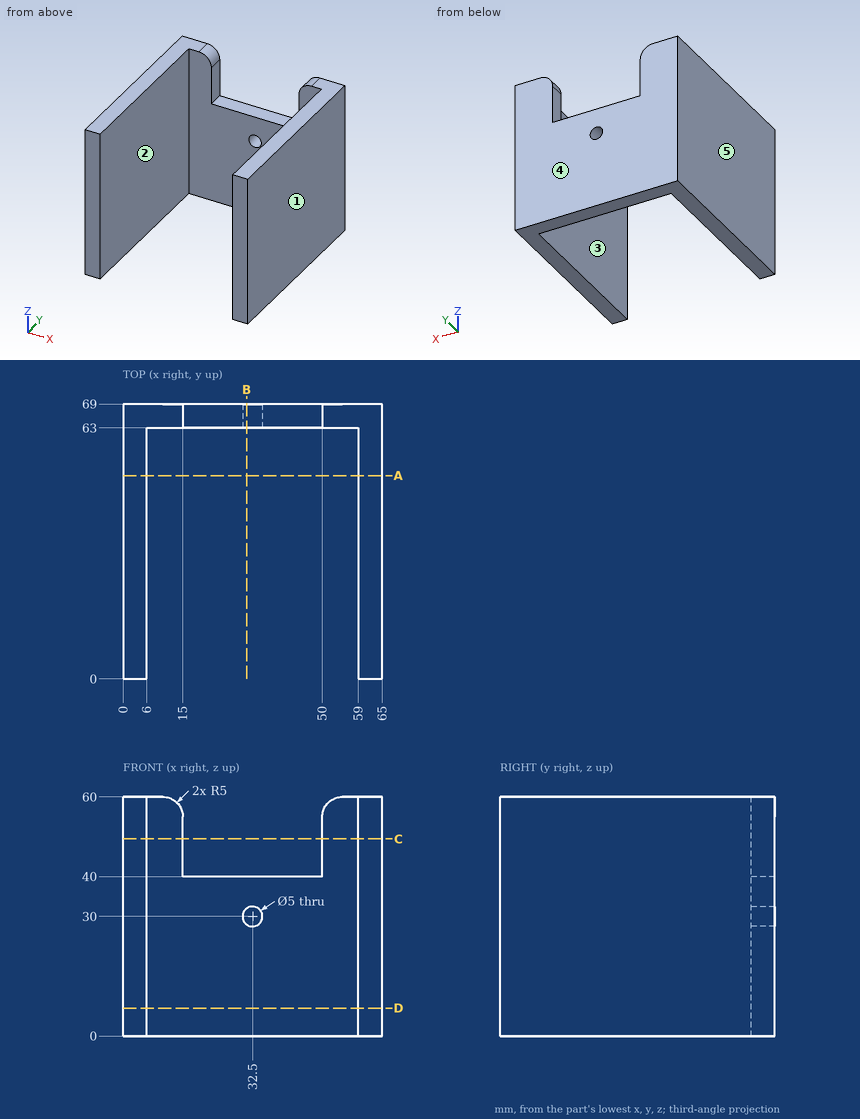
Here's the drawing with two shaded views (mm, measured from the low corner). I have some questions. A direction names the side the tool comes from. Round coordinates to 2 decimals unless told otherwise and drop trailing zeros. Loops run counter-clockwise (first coordinate to the right, second up) from the corner with the lowest first, then second, coordinate; pieces in that order, holes last.
Item 1: Suppose I cut it at C-C, the plane z = 49.5. Write out the boundary of the cut face in (x, y), then the cut area to 3 significant figures.
Item 2: Suppose I cut it at D-D, the plane z = 7. Write out the boundary of the cut face in (x, y).
Item 3: If we mould it in two halves opening along X, with no side actions, what happens to the marked faces 3, 4 and 5? For each: +X half, -X half, draft (parallel to the pull), parting line (faces both ways), or undercut.
Item 4: Which directions (+Z, -Z, +X, -X, +Y, -Y) give clear straight access to the entire face, cutting with the end or side of a thin tool? Please do the marked faces 1 and 2.
Item 5: Please list where these lines run through material, in increasing order: L1, parallel to X at y = 58.5, z = 28.5; L2, parallel to Z at x = 32.5, y = 65.9; L3, parallel to Y at x = 28, z = 38.
Item 6: Will these pins go through, and if not, where does the flat tip stop? pin 1 Ø16 at (x, z) = (25.5, 33.5) entering from -Y; pin 2 Ø1.8 at (x, y) = (34, 64.5) entering from +Z.
Item 7: Suppose I cut it at A-A, the plane y = 51. Write out the boundary of the cut face in (x, z).
Item 8: Suppose I cut it at B-B, the plane x = 31. Write out the boundary of the cut face in (y, z).
Reported:
1. outline: (0, 0) - (6, 0) - (6, 63) - (15, 63) - (15, 69) - (0, 69) - close; (50, 63) - (59, 63) - (59, 0) - (65, 0) - (65, 69) - (50, 69) - close
1. area: 936 mm2
2. outline: (0, 0) - (6, 0) - (6, 63) - (59, 63) - (59, 0) - (65, 0) - (65, 69) - (0, 69) - close
3. face 3: undercut
3. face 4: draft
3. face 5: -X half
4. face 1: +Z, -Z, +X, +Y, -Y
4. face 2: +Z, -Z, -Y
5. L1: x = 0 to 6, 59 to 65
5. L2: z = 0 to 27.5, 32.5 to 40
5. L3: y = 63 to 69
6. pin 1: stops at y = 63
6. pin 2: stops at z = 40
7. outline: (0, 0) - (6, 0) - (6, 60) - (0, 60) - close; (59, 0) - (65, 0) - (65, 60) - (59, 60) - close
8. outline: (63, 0) - (69, 0) - (69, 28) - (63, 28) - close; (63, 32) - (69, 32) - (69, 40) - (63, 40) - close
